Input: part model. Units: mm. Frame: model coordinates. A direction names the side the tool comes from. Round coordinates to 2 decimals unless told otherwise and drop trailing zeros. Write each loop counter-clockwise with the first axis right and the second up, starting at its lowest first coordinate (ties: lowest second). Pieces come first, ordered by that corner, then holes. Notation, with made-up numbers: M 48.25,15 L 79.25,15 A24 cw 79.25,46 Z; hole C 74,-32 d6. An arc over 180 degrees is marked long. Answer as CSV lines item,"result". Start each with the question number.
Autodesk Inventor part; units mm, degrees
ref_plane "작업 평면16" through (0, -21, 0) normal (0, 1, 0) x (-1, 0, 0)
ref_plane "YZ Plane" through (0, 0, 0) normal (1, 0, 0) x (0, 1, 0)
ref_plane "XY Plane" through (0, 0, 0) normal (0, 0, 1) x (1, 0, 0)
ref_plane "작업 평면16" through (0, -21, 0) normal (0, 1, 0) x (-1, 0, 0)
sketch "스케치46" plane through (0, -21, 0) normal (0, 1, 0) x (-1, 0, 0)
  spline S0 degree 3 poles (191.4874, -85.0161) (195.7231, -69.6387) (195.5194, -54.7481) (188.0983, -31.7262) (183.731, -23.2823) (177.7743, -15.0127) knots 0.143885 0.143885 0.143885 0.143885 0.581431 0.581431 0.843231 0.843231 0.843231 0.843231
  spline S1 degree 3 poles (189.2538, -92.0465) (190.1005, -89.6919) (190.845, -87.3484) (191.4874, -85.0161) knots 0.077523 0.077523 0.077523 0.077523 0.143885 0.143885 0.143885 0.143885
  arc A0 (183.4058, -96.885) -> (189.2538, -92.0465) centre (181.526, -88.6596) ccw
  spline S2 degree 3 poles (177.1168, -99.3875) (178.1345, -99.0781) (179.1243, -98.6874) (180.7924, -97.822) (181.4844, -97.3903) (182.1335, -96.8989) knots -0.627135 -0.627135 -0.627135 -0.627135 -0.308629 -0.308629 -0.063964 -0.063964 -0.063964 -0.063964
  ellipse E0 centre (180.8973, -97.418) end of major axis (175.52, -97.6575) minor radius 0.4767 (183.4058, -96.885) -> (182.1335, -96.8989) ccw
  spline S3 degree 3 poles (169.3014, -100.3265) (170.1206, -100.3155) (170.9637, -100.2934) (173.5928, -100.1416) (175.3872, -99.9134) (177.1168, -99.3875) knots -0.790866 -0.790866 -0.790866 -0.790866 -0.54231 -0.54231 0 0 0 0
  ellipse E1 centre (154.0427, -99.7705) end of major axis (172.6036, -100.1468) minor radius 0.4335 (166.2054, -100.3445) -> (169.3014, -100.3265) ccw
  line L0 (117.5358, -100.3445) -> (166.2054, -100.3445)
  spline S4 degree 3 poles (177.7743, -15.0127) (174.6367, -10.6567) (171.058, -6.3491) (167.0384, -2.0899) knots 0.843231 0.843231 0.843231 0.843231 0.981134 0.981134 0.981134 0.981134
  line L1 (167.0384, -2.0899) -> (104.9322, -2.0899)
  spline S5 degree 3 poles (104.9322, -2.0899) (102.452, -7.1506) (100.3104, -12.2796) (98.5075, -17.477) knots 0.836147 0.836147 0.836147 0.836147 1 1 1 1
  spline S6 degree 3 poles (98.5075, -17.477) (97.9178, -18.6748) (97.3597, -19.8935) (96.0924, -22.888) (95.4222, -24.6714) (94.4856, -27.5216) (94.1741, -28.5502) (93.7016, -30.2529) (93.5277, -30.9181) (93.2089, -32.2157) (93.0634, -32.8461) (92.745, -34.3177) (92.5794, -35.1581) (92.103, -37.8278) (91.8501, -39.6604) (91.6665, -41.4919) knots -2.526004 -2.526004 -2.526004 -2.526004 -2.120534 -2.120534 -1.544298 -1.544298 -1.220936 -1.220936 -1.014307 -1.014307 -0.819565 -0.819565 -0.560995 -0.560995 0 0 0 0
  line L2 (91.6665, -41.4919) -> (89.5894, -62.2122)
  spline S7 degree 3 poles (89.5894, -62.2122) (89.5894, -63.3351) (89.6133, -64.4561) (89.6986, -66.503) (89.7523, -67.4237) (89.8984, -69.389) (89.9946, -70.4286) (90.2978, -73.1917) (90.5351, -74.9036) (90.8157, -76.6062) knots -1.44821 -1.44821 -1.44821 -1.44821 -1.11115 -1.11115 -0.834292 -0.834292 -0.520567 -0.520567 0 0 0 0
  line L3 (90.8157, -76.6062) -> (94.465, -93.7314)
  arc A1 (94.465, -93.7314) -> (95.652, -93.9327) centre (165.2915, 320.1429) ccw
  ellipse E2 centre (105.5879, -87.8445) end of major axis (105.5879, -100.3445) minor radius 11.3766 (95.652, -93.9327) -> (96.6978, -95.6442) ccw
  arc A2 (96.6978, -95.6442) -> (98.3748, -96.4646) centre (98.7561, -93.561) ccw
  ellipse E3 centre (102.6075, -95.7007) end of major axis (109.3466, -95.2724) minor radius 0.6378 (98.3748, -96.4646) -> (99.6471, -96.4613) ccw
  spline S8 degree 3 poles (99.6471, -96.4613) (100.4112, -97.0879) (101.245, -97.6223) (103.148, -98.5885) (104.2178, -98.9855) (107.048, -99.7682) (109.0052, -100.0586) (111.2899, -100.1922) knots -1.504226 -1.504226 -1.504226 -1.504226 -1.123667 -1.123667 -0.686597 -0.686597 0 0 0 0
  spline S9 degree 3 poles (111.2899, -100.1922) (113.3488, -100.3126) (115.5027, -100.3445) (117.5358, -100.3445) knots -0.609915 -0.609915 -0.609915 -0.609915 0 0 0 0
  line L4 (117.5358, -100.3445) -> (166.2054, -100.3445)
  ellipse E4 centre (154.0427, -99.7705) end of major axis (172.6036, -100.1468) minor radius 0.4335 (166.2054, -100.3445) -> (169.3014, -100.3265) ccw
  spline S10 degree 3 poles (169.3014, -100.3265) (170.1206, -100.3155) (170.9637, -100.2934) (173.5928, -100.1416) (175.3872, -99.9134) (177.1168, -99.3875) knots -0.790866 -0.790866 -0.790866 -0.790866 -0.54231 -0.54231 0 0 0 0
  spline S11 degree 3 poles (177.1168, -99.3875) (178.1345, -99.0781) (179.1243, -98.6874) (180.7924, -97.822) (181.4844, -97.3903) (182.1335, -96.8989) knots -0.627135 -0.627135 -0.627135 -0.627135 -0.308629 -0.308629 -0.063964 -0.063964 -0.063964 -0.063964
  ellipse E5 centre (180.8973, -97.418) end of major axis (175.52, -97.6575) minor radius 0.4767 (183.4058, -96.885) -> (182.1335, -96.8989) ccw
  arc A3 (183.4058, -96.885) -> (189.2538, -92.0465) centre (181.526, -88.6596) ccw
  spline S12 degree 3 poles (189.2538, -92.0465) (190.1005, -89.6919) (190.845, -87.3484) (191.4874, -85.0161) knots 0.077523 0.077523 0.077523 0.077523 0.143885 0.143885 0.143885 0.143885
  spline S13 degree 3 poles (191.4874, -85.0161) (195.7231, -69.6387) (195.5194, -54.7481) (188.0983, -31.7262) (183.731, -23.2823) (177.7743, -15.0127) knots 0.143885 0.143885 0.143885 0.143885 0.581431 0.581431 0.843231 0.843231 0.843231 0.843231
  spline S14 degree 3 poles (189.5592, -84.485) (189.4545, -84.8653) (189.2663, -85.5314) (189.0415, -86.2939) (188.8686, -86.8664) (188.7513, -87.2483) (188.602, -87.7261) (188.4805, -88.1086) (188.326, -88.587) (188.2003, -88.9701) (188.0405, -89.4492) (187.9106, -89.8328) (187.7456, -90.3127) (187.5779, -90.7929) (187.441, -91.1774) (187.3718, -91.3698) knots 0.077523 0.077523 0.077523 0.077523 0.088583 0.096878 0.099644 0.105174 0.107939 0.113469 0.116234 0.121764 0.124529 0.130059 0.132824 0.138354 0.143885 0.143885 0.143885 0.143885
  arc A4 (180.8973, -95.3262) -> (187.3718, -91.3698) centre (181.2393, -88.61) ccw
  spline S15 degree 3 poles (180.8973, -95.3262) (180.6943, -95.4789) (180.3216, -95.7405) (179.8747, -96.018) (179.5233, -96.221) (179.2849, -96.3513) (178.9819, -96.5081) (178.7361, -96.6283) (178.4248, -96.7723) (178.1725, -96.8825) (177.8532, -97.0141) (177.5947, -97.1146) (177.268, -97.2343) (176.9377, -97.3481) (176.6698, -97.433) (176.535, -97.474) knots -0.622898 -0.622898 -0.622898 -0.622898 -0.533273 -0.462877 -0.439411 -0.39248 -0.369015 -0.322084 -0.298619 -0.251688 -0.228222 -0.181292 -0.157826 -0.110895 -0.063964 -0.063964 -0.063964 -0.063964
  line L5 (176.535, -97.474) -> (111.4067, -98.1956)
  spline S16 degree 3 poles (111.4067, -98.1956) (111.0082, -98.1723) (110.2355, -98.1159) (109.3273, -98.0206) (108.4602, -97.9064) (107.7985, -97.7999) (107.0879, -97.6629) (106.6323, -97.562) (106.2272, -97.4625) (106.0103, -97.4058) (105.7968, -97.3472) (105.6552, -97.307) (105.3736, -97.224) (105.0254, -97.1142) (104.5121, -96.935) (104.1099, -96.7784) (103.7148, -96.6109) (103.455, -96.4936) (103.1348, -96.3398) (102.8824, -96.2109) (102.573, -96.043) (102.3302, -95.9032) (101.9734, -95.685) (101.5109, -95.3793) (101.1273, -95.0886) (100.9153, -94.9147) knots 0 0 0 0 0.125352 0.250704 0.31338 0.438733 0.501409 0.595423 0.626761 0.673768 0.689437 0.720775 0.736444 0.814789 0.877465 0.971479 1.002817 1.065493 1.096832 1.159508 1.190846 1.253522 1.28486 1.378874 1.504226 1.504226 1.504226 1.504226
  arc A5 (96.293, -91.0501) -> (100.9153, -94.9147) centre (102.2083, -88.6716) ccw
  arc A6 (92.3068, -61.3872) -> (96.293, -91.0501) centre (227.7562, -58.2846) ccw
  arc A7 (107.3313, -4.0899) -> (92.3068, -61.3872) centre (218.4178, -63.8374) ccw
  line L6 (107.3313, -4.0899) -> (166.1723, -4.0899)
  spline S17 degree 3 poles (166.1723, -4.0899) (166.7932, -4.7558) (167.8603, -5.9228) (169.041, -7.2601) (169.91, -8.2645) (170.4809, -8.9348) (171.1843, -9.7736) (171.7386, -10.4454) (172.4212, -11.286) (172.959, -11.9593) (173.6208, -12.8017) (174.142, -13.4764) (174.7831, -14.3207) (175.4139, -15.1658) (175.9075, -15.8429) (176.1515, -16.1817) knots 0.843231 0.843231 0.843231 0.843231 0.865071 0.881452 0.886912 0.897832 0.903292 0.914212 0.919672 0.930592 0.936052 0.946972 0.952432 0.963352 0.974272 0.974272 0.974272 0.974272
  spline S18 degree 3 poles (176.1515, -16.1817) (177.4538, -17.9897) (179.9013, -21.6192) (182.5692, -26.1898) (184.9446, -30.7857) (186.6116, -34.4828) (188.4049, -39.1304) (189.6076, -42.8697) (190.8225, -47.5717) (191.5638, -51.3563) (192.2029, -56.1175) (192.4844, -59.9515) (192.5489, -64.7775) (192.3706, -68.6656) (191.8595, -73.5618) (191.0598, -78.4947) (190.1111, -82.4814) (189.5592, -84.485) knots 0.143885 0.143885 0.143885 0.143885 0.202163 0.260442 0.289582 0.347861 0.377 0.435279 0.464418 0.522697 0.551837 0.610116 0.639255 0.697534 0.726673 0.784952 0.843231 0.843231 0.843231 0.843231
  circle A8 centre (157.0041, -93.6029) radius 2.75
  circle A9 centre (157.0041, -93.6029) radius 4.75
  line L7 (176.535, -97.474) -> (111.4067, -98.1956)
  circle A10 centre (164.2713, -9.3093) radius 2.75
  circle A11 centre (164.2713, -9.3093) radius 4.75
  circle A12 centre (110.4218, -9.3093) radius 2.75
  circle A13 centre (110.4218, -9.3093) radius 4.75
  line L8 (154.2569, -58.8887) -> (127.2569, -58.8887)
  line L9 (127.2569, -58.8887) -> (127.2569, -39.3887)
  line L10 (154.2569, -39.3887) -> (154.2569, -58.8887)
  line L11 (146.7569, -39.3887) -> (146.7569, -36.3887)
  line L12 (146.7569, -36.3887) -> (134.7569, -36.3887)
  line L13 (134.7569, -36.3887) -> (134.7569, -39.3887)
  line L14 (127.2569, -39.3887) -> (134.7569, -39.3887)
  line L15 (146.7569, -39.3887) -> (154.2569, -39.3887)
  line L16 (121.2569, -62.8887) -> (160.2569, -62.8887)
  line L17 (160.2569, -62.8887) -> (160.2569, -34.8887)
  line L18 (160.2569, -34.8887) -> (121.2569, -34.8887)
  line L19 (121.2569, -34.8887) -> (121.2569, -62.8887)
  line L20 (162.2569, -64.8887) -> (119.2569, -64.8887)
  line L21 (119.2569, -64.8887) -> (119.2569, -32.8887)
  line L22 (119.2569, -32.8887) -> (162.2569, -32.8887)
  line L23 (162.2569, -32.8887) -> (162.2569, -64.8887)
  line L24 (136.7569, -62.8887) -> (136.7569, -64.8887)
  line L25 (144.7569, -62.8887) -> (144.7569, -64.8887)
  line L26 (140.7569, -58.8887) -> (140.7569, -78.8674)
  point P0 (0, 0)
  point P1 (135.3739, -0.3445)
  point P2 (177.7743, -15.0127)
  point P3 (159.4693, -97.6631)
  point P4 (154.6295, -97.7167)
  dimension "d272" = 5.5
  dimension "d273" = 2
  dimension "d274" = 5.5
  dimension "d275" = 2
  dimension "d276" = 5.5
  dimension "d277" = 2
  dimension "d284" = 27
  dimension "d285" = 19.5
  dimension "d286" = 12
  dimension "d287" = 7.5
  dimension "d288" = 3
  dimension "d291" = 3
  dimension "d292" = 39
  dimension "d293" = 28
  dimension "d294" = 6
  dimension "d295" = 4
  dimension "d296" = 2
  dimension "d297" = 4
  dimension "d298" = 4
extrude "돌출51" add sketch "스케치46" along normal blind 3 contours S1 A0 E0 S2 S3 E1 L0 S9 S8 E3 A2 E2 A1 L3 S7 L2 S6 S5 L1 S4 S0 | S14 A4 S15 L5 A9 S16 A5 A6 A7 L6 S17 S18 | A9 L5 | L5 A9 | A8 | A10 | A11 | A12 | A13 | L16 L19 L18 L17 | L16 L25 L20 L26 | L26 L20 L24 L16 | L8 L9 L14 L13 L12 L11 L15 L10 | L24 L20 L21 L22 L23 L25 L16 L17 L18 L19
extrude "돌출53" add sketch "스케치46" against normal blind 7 contours A9 L5 | L5 A9 | A11 | A13
extrude "돌출54" cut sketch "스케치46" along normal blind 7 contours L8 L9 L14 L13 L12 L11 L15 L10
extrude "돌출55" add sketch "스케치46" against normal blind 3 contours L24 L20 L21 L22 L23 L25 L16 L17 L18 L19
properties part number "장갑_위_찐"
Item 1: Access query for faces 1 (the face through (-142, -20, -100.344)), 2 (the face through (-139.1, -24, -34.6)), 3 (the face through (-160.257, -22, -49)), 4 (the face through (-154.257, -20, -49)), 5 (the face through (-112.5, -28, -11.4)). Directions: +Z, -Z, +X, -X, +Y, -Y. A direction counts if a zero-diameter tool reaches every point of the face in a straight line with its end or side. Return the directions, or none.
Item 2: Pin query (flat end, axial travel): pin 1 Ø2.5 at (x, y) = (-150, -23) entering from +Z; pin 2 Ø0.9 at (y, z) = (-22.5, -53.5) entering from +X; pin 3 Ø0.9 at (y, z) = (-19, -50) entering from -X; pin 4 Ø2 at (y, z) = (-23, -31.5) entering from +X. Return the tip coordinate at first contact, or that it passes through.
Item 3: Line query: line 1 (X direction, y = -23.25, z = -44.5); line 2 (Y direction, x = -104.5, z = -89.5); line 3 (Z direction, x = -124.5, y = -22.25). Output: solid intervals per line, ascending. Write a range as [from, to].
Item 4: Draft query along Z for faces 6 (the face through (-129, -22, -62.889)), 7 (the face through (-90.642, -19.521, -51.707)), 8 (the face through (-119.257, -22, -49)), 9 (the face through (-92.615, -19.521, -85.049)). Return one class per face: +Z half, -Z half, draft (parallel to the pull), parting line (faces both ways), or undercut.
Item 5: Cut plane A-A, the plane x = -132. Return loops of the section in (y, z).
Item 6: Cut plane B-B, the plane y = -26. Return loops of the section in (x, z), plus the area to 3 significant figures.
Results list:
1,face 1,"-Z, +X, -X, +Y, -Y"
1,face 2,"+X, -X, -Y"
1,face 3,"-Y"
1,face 4,"+Y, -Y"
1,face 5,"+Z, -Z, +X, -X, -Y"
2,pin 1,"z = -32.89"
2,pin 2,"x = -119.26"
2,pin 3,"x = -193.39"
2,pin 4,"through"
3,line 1,"[-162.26, -160.26], [-121.26, -119.26]"
3,line 2,"[-21, -18]"
3,line 3,"[-64.89, -62.89], [-34.89, -32.89]"
4,face 6,"undercut"
4,face 7,"+Z half"
4,face 8,"draft"
4,face 9,"-Z half"
5,outline,"M -24,-64.89 L -21,-64.89 L -21,-100.34 L -18,-100.34 L -18,-58.89 L -21,-58.89 L -21,-62.89 L -24,-62.89 Z; M -24,-34.89 L -21,-34.89 L -21,-39.39 L -18,-39.39 L -18,-2.09 L -21,-2.09 L -21,-32.89 L -24,-32.89 Z"
6,outline,"C -164.27,-9.31 d9.5; C -157,-93.6 d9.5; C -110.42,-9.31 d9.5; hole C -164.27,-9.31 d5.5; hole C -157,-93.6 d5.5; hole C -110.42,-9.31 d5.5"
6,area,"141 mm²"
